For this review, take the finished solid that the model builds, in its own axes (mm). Face numbers are marked on the shaded views. A direction names the side the tool comes from. Round coordinates to 2 decimals unless told otherwise and drop trailing zeros. Loops run counter-clockwise (first coordinate to the right, second up) from the corner with the lowest first, then second, coordinate; pieces in that order, holes last. Notation, with made-up numbers: (1, 7.25) -> (14, 7.25) arc R29 ccw to (14, 29.25) -> close; hole circle Ø5 at (13, 18.5). An arc over 180 degrees is marked (long way). Write each question's results on one line, items separated by ' | '.
Autodesk Inventor part; units mm, degrees
ref_plane "YZ Plane" through (0, 0, 0) normal (1, 0, 0) x (0, 1, 0)
ref_plane "XZ Plane" through (0, 0, 0) normal (0, 1, 0) x (-1, 0, 0)
ref_plane "XY Plane" through (0, 0, 0) normal (0, 0, 1) x (1, 0, 0)
sketch "Sketch1" plane through (0, 0, 0) normal (0, 1, 0) x (-1, 0, 0)
  line L0 (-19, -3.5) -> (-19, 3.5)
  line L1 (-19, 3.5) -> (19, 3.5)
  line L2 (19, 3.5) -> (19, -3.5)
  line L3 (19, -3.5) -> (-19, -3.5)
  line L4 (-19, -3.5) -> (19, 3.5) construction
  line L5 (-19, 3.5) -> (19, -3.5) construction
  circle A0 centre (19, 0) radius 1.5
  line L6 (19, 3.5) -> (22.5, 3.5)
  line L7 (22.5, 3.5) -> (22.5, -3.5)
  line L8 (22.5, -3.5) -> (19, -3.5)
  line L9 (19, -3.5) -> (19, 3.5)
  line L10 (-19, 0) -> (-19, -7.8)
  line L11 (-22.5, 14.8) -> (-22.5, -7.8)
  line L12 (-22.5, -7.8) -> (-15.5, -7.8)
  line L13 (-15.5, -7.8) -> (-15.5, 14.8)
  line L14 (-15.5, 14.8) -> (-22.5, 14.8)
  line L15 (-22.5, 14.8) -> (-15.5, -7.8) construction
  line L16 (-22.5, -7.8) -> (-15.5, 14.8) construction
  line L17 (-19, 3.5) -> (-22.5, 3.5)
  circle A1 centre (-19, -7.8) radius 1.5
  line L18 (-15.5, -7.8) -> (-22.5, -7.8)
  line L19 (-22.5, -7.8) -> (-22.5, -11.3)
  line L20 (-22.5, -11.3) -> (-15.5, -11.3)
  line L21 (-15.5, -11.3) -> (-15.5, -7.8)
  point P0 (0, 0)
  point P1 (-22.5, -7.8)
  point P2 (-15.5, -3.5)
  dimension "d0" = 7
  dimension "d1" = 38
  dimension "d2" = 3
  dimension "d3" = 3.5
  dimension "d4" = 7.8
  dimension "d5" = 7
  dimension "d6" = 3
  dimension "d7" = 3.5
extrude "Extrusion1" add sketch "Sketch1" along normal blind 5 contours L10 A1 L12 L11 L17 L0 | L0 L1 L13 L3 | L3 L13 L12 A1 L10 | L13 L1 L2 A0 L3 | L2 A0 L6 L7 L8 | L21 L20 L19 L12 A1
fillet "Fillet1" radius 3.5 5 edges at (22.5, 2.5, -11.3) (15.5, 2.5, -11.3) (22.5, 2.5, 3.5) (-22.5, 2.5, 3.5) (-22.5, 2.5, -3.5)
sketch "Sketch2" plane through (0, 5, 0) normal (0, 1, 0) x (1, 0, 0)
  arc A0 (19, -3.5) -> (22.5, 0) centre (19, 0) ccw
  line L0 (22.5, 0) -> (64, 0)
  line L1 (15.5, 3.5) -> (22.5, 3.5)
  line L2 (22.5, 3.5) -> (22.5, -3.5)
  line L3 (22.5, -3.5) -> (15.5, -3.5)
  line L4 (15.5, -3.5) -> (15.5, 3.5)
  line L5 (22.5, -3.5) -> (64, -3.5)
  line L6 (64, -3.5) -> (64, 3.5)
  line L7 (64, 3.5) -> (22.5, 3.5)
  line L8 (22.5, 3.5) -> (22.5, -3.5)
  line L9 (64, 3.5) -> (67.5, 3.5)
  line L10 (67.5, 3.5) -> (67.5, -3.5)
  line L11 (67.5, -3.5) -> (64, -3.5)
  line L12 (64, -3.5) -> (64, 3.5)
  circle A1 centre (64, 0) radius 1.65
  point P0 (0, 0)
  point P1 (22.5, 0)
  point P2 (19, -3.5)
  dimension "d11" = 41.5
  dimension "d12" = 3.5
  dimension "d13" = 3.3
extrude "Extrusion2" add sketch "Sketch2" against normal up to surface (5 mm away) contours A0 L2 L3 | L2 L7 L6 A1 L0 | L0 A1 L6 L5 L2 | L6 A1 L9 L10 L11
fillet "Fillet2" radius 3.5 2 edges at (67.5, 2.5, 3.5) (67.5, 2.5, -3.5)
sketch "Sketch3" plane through (0, 5, 0) normal (0, 1, 0) x (1, 0, 0)
  line L0 (19, 0) -> (57, 0)
  line L1 (19, 0) -> (60.5, 0)
  line L2 (19, 0) -> (60.5, 0) construction
  circle A0 centre (60.5, 0) radius 1.65
  point P0 (0, 0)
  dimension "d17" = 38
  dimension "d18" = 41.5
  dimension "d19" = 0
  dimension "d20" = 3.3
extrude "Extrusion3" cut sketch "Sketch3" against normal blind 10
sketch "Sketch4" plane through (0, 5, 0) normal (0, 1, 0) x (1, 0, 0)
  line L0 (-19, -3.5) -> (64, -3.5)
  line L1 (62.2745, -3.5) -> (67.2267, -3.5)
  line L2 (67.2267, -3.5) -> (67.2267, 3.993)
  line L3 (67.2267, 3.993) -> (62.2745, 3.993)
  line L4 (62.2745, 3.993) -> (62.2745, -3.5)
  line L5 (67.2267, 3.993) -> (67.8067, 3.993)
  line L6 (67.8067, 3.993) -> (67.8067, -3.5)
  line L7 (67.8067, -3.5) -> (67.2267, -3.5)
  line L8 (67.2267, -3.5) -> (67.2267, 3.993)
  point P0 (0, 0)
extrude "Extrusion4" cut sketch "Sketch4" against normal blind 10
sketch "Sketch5" plane through (0, 5, 0) normal (0, 1, 0) x (1, 0, 0)
  circle A0 centre (60.5, 0) radius 1.65
  line L0 (60.5, 0) -> (64, 0)
  line L1 (-19, -3.5) -> (62.2745, -3.5)
  line L2 (60.5, -3.5) -> (64, -3.5)
  line L3 (64, -3.5) -> (64, 3.5)
  line L4 (64, 3.5) -> (60.5, 3.5)
  line L5 (60.5, 3.5) -> (60.5, -3.5)
  point P0 (0, 0)
  point P1 (60.5, 1.65)
  point P2 (60.5, -1.65)
  dimension "d25" = 3.5
  dimension "d26" = 7
extrude "Extrusion5" add sketch "Sketch5" against normal up to surface (5 mm away) contours L0 L3 L2 L1 L5 A0 | A0 L5 L4 L3 L0
fillet "Fillet3" radius 3.5 2 edges at (64, 2.5, 3.5) (64, 2.5, -3.5)
sketch "Sketch6" plane through (0, 5, 0) normal (0, 1, 0) x (1, 0, 0)
  circle A0 centre (19, 7.8) radius 1.5
  line L0 (19, 7.8) -> (19, 0)
  circle A1 centre (-19, 0) radius 1.5
  line L1 (19, 0) -> (-19, 0)
  line L2 (-19, 0) -> (19, 0)
  line L3 (19, 0) -> (57, 0)
  line L4 (60.5, 3.5) -> (22.5, 3.5)
  line L5 (57, 3.5) -> (64.573, 3.5)
  line L6 (64.573, 3.5) -> (64.573, -3.5)
  line L7 (64.573, -3.5) -> (57, -3.5)
  line L8 (57, -3.5) -> (57, 3.5)
  point P0 (0, 0)
  dimension "d30" = 38
extrude "Extrusion6" add sketch "Sketch6" against normal up to surface (5 mm away) contours L5 L6 L7 L8 L4
sketch "Sketch7" plane through (0, 5, 0) normal (0, 1, 0) x (1, 0, 0)
  circle A0 centre (19, 7.8) radius 1.5
  line L0 (19, 7.8) -> (19, 0)
  line L1 (19, 0) -> (57, 0)
  circle A1 centre (57, 0) radius 1.5
  line L2 (57, 0) -> (60.5, 0)
  line L3 (-19, -3.5) -> (64.573, -3.5)
  line L4 (64.573, 3.5) -> (22.5, 3.5)
  line L5 (60.5, -3.5) -> (64.573, -3.5)
  line L6 (64.573, -3.5) -> (64.573, 3.5)
  line L7 (64.573, 3.5) -> (60.5, 3.5)
  line L8 (60.5, 3.5) -> (60.5, -3.5)
  point P0 (0, 0)
  point P1 (64.573, -3.5)
  dimension "d33" = 7.8
  dimension "d34" = 38
  dimension "d35" = 3
  dimension "d36" = 3.5
extrude "Extrusion7" cut sketch "Sketch7" against normal blind 10 contours A1 L2 L1 | L1 L2 A1 | L8 L4 L6 L3
fillet "Fillet4" radius 3.5 2 edges at (60.5, 2.5, -3.5) (60.5, 2.5, 3.5)
properties part number "connector"
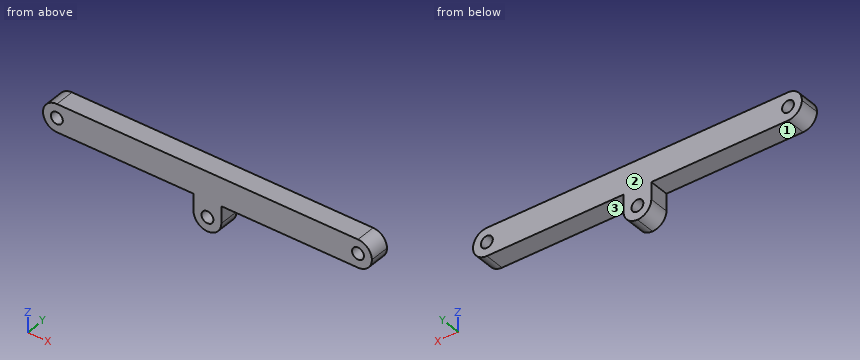
1. To check wall thickness, follow probe 1 along X at (y, z) = (2.3, 0); probe 2 along X at (y, z) = (3.8, -7.8); probe 3 along X at (y, z) = (0.5, -1). State the ranges of each line that lie inside material, in increasing order.
Values found:
probe 1: x = -22.5 to -20.5, -17.5 to 55.5, 58.5 to 60.5 | probe 2: x = 15.5 to 17.5, 20.5 to 22.5 | probe 3: x = -22.35 to -20.12, -17.88 to 55.88, 58.12 to 60.35
2. Consider section B-B (z = -7). State the section outline as (x, y) points, plus the area to 3 significant figures.
Values found:
outline: (15.5, 0) -> (17.73, 0) -> (17.73, 5) -> (15.5, 5) -> close; (20.27, 0) -> (22.5, 0) -> (22.5, 5) -> (20.27, 5) -> close | area: 22.3 mm2
3. For pin 1 (2.5 mm diameter, centred on x = 57, z = 0, fed in from -Y); pin 2 (2 mm diameter, centred on x = 49.5, y = 3.5, fed in from -Z); pin 3 (3.5 mm diameter, centred on x = 19, z = -7.8, fed in from +Y); pin 4 (2 mm diameter, centred on y = 2.5, z = -5, fed in from +X), all flat-tipped, find the tip position at first contact; note any pin that passes through.
Values found:
pin 1: passes through | pin 2: stops at z = -3.5 | pin 3: stops at y = 5 | pin 4: stops at x = 22.5
4. Tool access review of the marked faces 1, 2 and 3: name each direction out of +Z, -Z, +X, -X, +Y, -Y from which nothing blocks a thin tool from reaching the whole face with its end or side.
Values found:
face 1: -Z, -X, +Y, -Y | face 2: +Z, -Z, +X, -X, +Y | face 3: -Z, +X, +Y, -Y
5. Consider section A-A (y = 2.4). Give the number of separate pieces and of enclosed holes in the cut face, plus the area to 3 significant figures.
Values found:
separate pieces: 1 | enclosed holes: 3 | area: 599 mm2
6. Consider section C-C (x = 42). State the section outline as (y, z) points, plus the area to 3 significant figures.
Values found:
outline: (0, -3.5) -> (5, -3.5) -> (5, 3.5) -> (0, 3.5) -> close | area: 35.0 mm2
